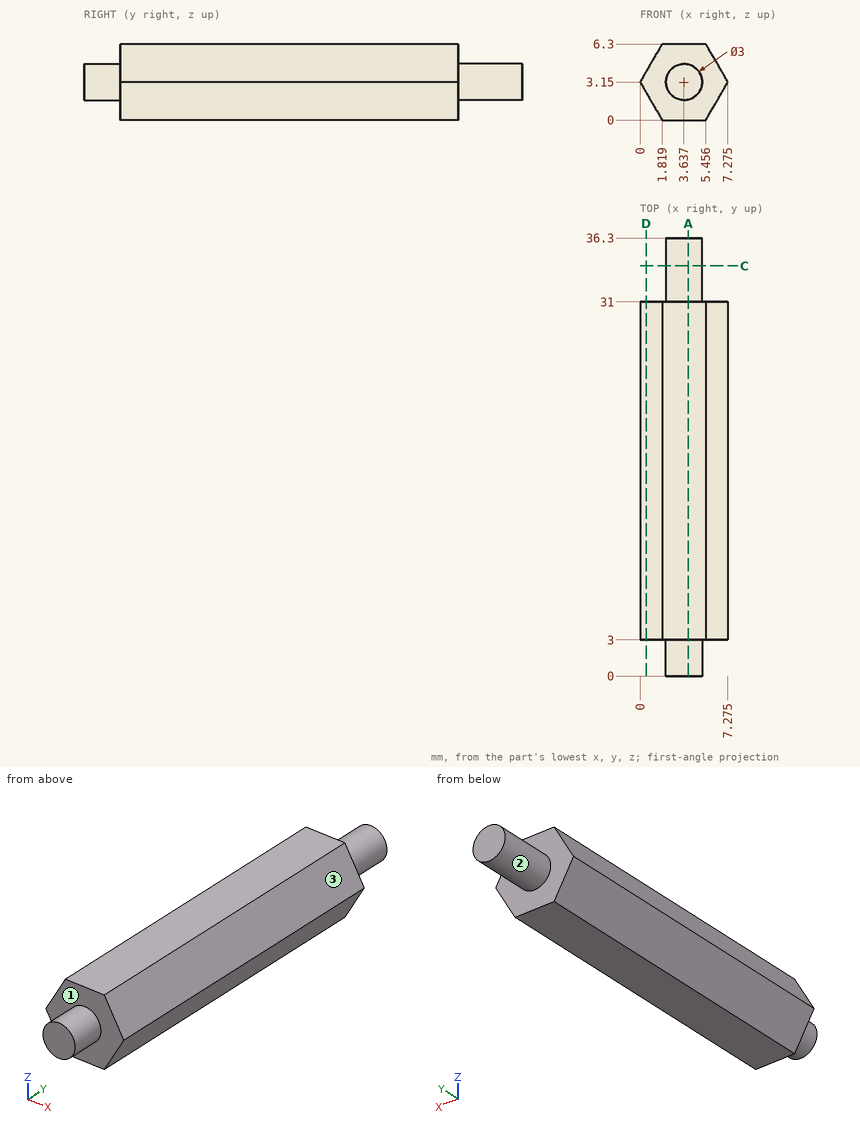
Source: three-view drawing plus pictorial views. Frame: mm from the lowest corner of the part. A direction names the side the tool comes from. Give positions to 0.01 mm unless a question says otherwise; leave off trailing zeros. Write each loop counter-clockwise with the first axis right and the second up, starting at its lowest first coordinate (ties: lowest second). Pieces come first, ordered by that corner, then holes. Notation, with made-up numbers: (-38.5, 59.5) - (15.5, 59.5) arc R22 cw to (15.5, 73.5) - close; hole circle Ø7 at (-9.5, 19). An arc over 180 degrees is marked (long way). Write item = value, one per line. Start each with the question number.
1. First-contact query: pin 1 Ø1.5 at (y, z) = (18.5, 2) entering from +X. Flat tip, straight axial feed; report the tip coordinate or a pass-through.
2. Section query A-A, the plane x = 4. Output: boundary loops of the cut face in (y, z) (1 decimal).
3. Access query for the marked faces 1, 2 and 3. Directions: +Z, -Z, +X, -X, +Y, -Y. A direction counts if a zero-diameter tool reaches every point of the face in a straight line with its end or side. Return the directions, or none.
4. Section query D-D, the plane x = 0.5. Output: boundary loops of the cut face in (y, z), then the cut area to 3 significant figures.
5. Section query C-C, the plane y = 34. Output: boundary loops of the cut face in (x, z).
6. Ray query, L1, parallel to Y at x = 2, z = 2.5; L2, parallel to X at y = 11.5, z = 3 (1 decimal); L3, parallel to X at y = 6.5, z = 2.25 (1 decimal). Return the intervals inside material, ascending.
Check sheet entries:
q1.pin_1 = 7.04
q2.outline = (0, 1.7) - (3, 1.7) - (3, 0) - (31, 0) - (31, 1.7) - (36.3, 1.7) - (36.3, 4.6) - (31, 4.6) - (31, 6.3) - (3, 6.3) - (3, 4.6) - (0, 4.6) - close
q3.face_1 = -Y
q3.face_2 = +Y
q3.face_3 = +Z, +X, +Y, -Y
q4.outline = (3, 2.28) - (31, 2.28) - (31, 4.02) - (3, 4.02) - close
q4.area = 48.5 mm2
q5.outline = circle Ø3 at (3.64, 3.15)
q6.L1 = 3 to 31
q6.L2 = 0.1 to 7.2
q6.L3 = 0.5 to 6.8
